```python
from build123d import *

# Parameters (mm, degrees)
F0_R     = 75
F1_DEPTH = 80
F2_R     = 5
F3_R     = 5
F4_DEPTH = 80


with BuildPart() as f1:
    # F0 (on Top) → F1 (new body)
    with BuildSketch(Plane.XY):
        Circle(F0_R)
    extrude(amount=F1_DEPTH)

    # F2
    f2_edges = [f1.edges().sort_by_distance(p)[0] for p in [
        (-75, 0, 80),
    ]]
    fillet(f2_edges, radius=F2_R)

    # F3 (on face) → F4 (cut, through all)
    with BuildSketch(Plane.XY.offset(80)):
        with Locations((-17.67767, 17.67767)):
            Circle(F3_R)
        with Locations((0, 25)):
            Circle(F3_R)
        with Locations((17.67767, 17.67767)):
            Circle(F3_R)
        with Locations((25, 0)):
            Circle(F3_R)
        with Locations((0, -25)):
            Circle(F3_R)
        with Locations((17.67767, -17.67767)):
            Circle(F3_R)
        with Locations((-17.67767, -17.67767)):
            Circle(F3_R)
        with Locations((-25, 0)):
            Circle(F3_R)
    extrude(amount=-F4_DEPTH, mode=Mode.SUBTRACT)


solid = f1.part
```
Source: CAD feature listing. Evaluate the final solid. Frame: model axes, mm. Coordinates: 2 decimals unless noted, no trailing zeros. Write each loop counter-clockwise with the first axis right and the second up, starting at its lowest first coordinate (ties: lowest second). Pieces come first, ordered by that corner, then holes. Notation, with made-up numbers: (59.25, 79) -> (100.25, 79) arc R19 cw to (100.25, 112) -> close; hole circle Ø8 at (-8, -21). An arc over 180 degrees is marked (long way). Return JSON: item names as keys, results as strings. Group by question number.
1) Section query C-C, the plane z = 59.5. State how many separate pieces and enclosed holes the cut face has, plus the area to 3 significant figures.
2) Ray query, line 1 along X through (y, z) = (-19, 21); line 2 along Y through (x, z) = (-2, 36.5); line 3 along Y through (x, z) = (24, 68). Return the intervals inside material, ascending.
3) Contact query for flat-ended pins moving along their axis: P1, Ø3, axis at y = -8, z = 52, coming from the -X side; P2, Ø9, axis at x = -17.68, y = -17.68, coming from the -Z side; P3, Ø8, axis at y = 46, z = 50, coming from the -X side; P4, Ø4, axis at x = 33.5, z = 20.5, coming from the +Y side. Output: stop coordinate, or through.
4) Mould query, pull axis Y, two halves, no side actions, for faces 1 (the face through (-1.08, -29.88, 40.56)), 2 (the face through (-9.764, 74.362, 36.975)), 3 (the face through (-1, 1, 80)). Classes: +Y half, -Y half, draft (parallel to the pull), parting line (faces both ways), or undercut.
5) Section query A-A, the plane y = 0. Return loops of the section in (x, z), plus the area to 3 significant figures.
From the geometry:
{
 "1": {"separate pieces": "1", "enclosed holes": "8", "area": "17,000 mm²"},
 "2": {"line 1": "-72.55 to -22.5, -12.86 to 12.86, 22.5 to 72.55", "line 2": "-74.97 to -29.58, -20.42 to 20.42, 29.58 to 74.97", "line 3": "-71.06 to -4.9, 4.9 to 71.06"},
 "3": {"P1": "x = -74.72", "P2": "through", "P3": "x = -62.14", "P4": "y = 68.06"},
 "4": {"face 1": "undercut", "face 2": "parting line", "face 3": "draft"},
 "5": {"outline": "(-75, 0) -> (-30, 0) -> (-30, 80) -> (-70, 80) arc R5 ccw to (-75, 75) -> close; (-20, 0) -> (20, 0) -> (20, 80) -> (-20, 80) -> close; (30, 0) -> (75, 0) -> (75, 75) arc R5 ccw to (70, 80) -> (30, 80) -> close", "area": "10,400 mm²"}
}
